Read the model definition and answer for the solid it produces. Units are mm, in the model's axes. A direction names the side the tool comes from. Coordinates: 2 decimals unless noted, no trailing zeros. Write each loop counter-clockwise with the first axis right and the second up, starting at its lowest first coordinate (ties: lowest second). Pieces come first, ordered by that corner, then holes. Notation, with made-up numbers: M 18.5,5.25 L 53.5,5.25 A18 ccw 53.5,39.25 Z; hole C 87.25,23 d7. An arc over 180 degrees is marked long. Write item = value, one per line.
from build123d import *

# Parameters (mm, degrees)
BOSS_EXTRUDE1_DEPTH = 14
SKETCH2_R           = 2
CUT_EXTRUDE1_DEPTH  = 20
SKETCH3_R           = 3.5
CUT_EXTRUDE2_DEPTH  = 3
SKETCH4_R           = 2.5
CUT_EXTRUDE3_DEPTH  = 8
FILLET1_R           = 0.5


with BuildPart() as part:
    # Sketch1 → Boss-Extrude1 (new body)
    with BuildSketch(Plane(origin=(0, 0, 0), x_dir=(1, 0, 0), z_dir=(0, 1, 0))):
        with BuildLine():
            Line((9, -14), (21, -14))
            Line((21, -14), (21, -20))
            Line((21, -20), (-21, -20))
            Line((-21, -20), (-21, -14))
            Line((-21, -14), (-9, -14))
            Line((-9, -14), (-9, 12.8))
            Line((-9, 12.8), (-1, 12.8))
            Line((-1, 12.8), (-1, 3.872983346))
            ThreePointArc((-1, 3.872983346), (0, -4), (1, 3.872983346))
            Line((1, 3.872983346), (1, 12.8))
            Line((1, 12.8), (9, 12.8))
            Line((9, 12.8), (9, -14))
        make_face()
    extrude(amount=BOSS_EXTRUDE1_DEPTH)

    # Sketch2 → Cut-Extrude1 (cut)
    with BuildSketch(Plane(origin=(9, 0, 0), x_dir=(0, 0, -1), z_dir=(1, 0, 0))):
        with Locations((8.3, 7)):
            Circle(SKETCH2_R)
    extrude(amount=-CUT_EXTRUDE1_DEPTH, mode=Mode.SUBTRACT)

    # Sketch3 → Cut-Extrude2 (cut)
    with BuildSketch(Plane(origin=(9, 0, 0), x_dir=(0, 0, -1), z_dir=(1, 0, 0))):
        with Locations((8.3, 7)):
            Circle(SKETCH3_R)
    extrude(amount=-CUT_EXTRUDE2_DEPTH, mode=Mode.SUBTRACT)

    # Sketch4 → Cut-Extrude3 (cut)
    with BuildSketch(Plane.XY.offset(20)):
        with Locations((-16, 7)):
            Circle(SKETCH4_R)
        with Locations((16, 7)):
            Circle(SKETCH4_R)
    extrude(amount=-CUT_EXTRUDE3_DEPTH, mode=Mode.SUBTRACT)

    # Fillet1
    fillet1_edges = [part.edges().sort_by_distance(p)[0] for p in [
        (-21, 7, 14),
        (-9, 7, 14),
        (-9, 7, -12.8),
        (9, 7, -12.8),
        (9, 7, 14),
        (21, 7, 14),
        (21, 7, 20),
        (-21, 7, 20),
    ]]
    fillet(fillet1_edges, radius=FILLET1_R)


solid = part.part
Item 1: Find section B-B (x = 16). Determine the outline of the cut face in (y, z).
Worked answers:
outline = M 0,14 L 4.5,14 L 4.5,20 L 0,20 Z; M 9.5,14 L 14,14 L 14,20 L 9.5,20 Z
Item 2: Consider line 1 along X through (y, z) = (4.75, 14.5); line 2 along Y through (x, z) = (16, 16.6); line 3 along X through (y, z) = (9, 12). Determine where each line is inside the solid, lowest interval first. Write a range as from..to.
Worked answers:
line_1 = -21..-17.09, -14.91..14.91, 17.09..21
line_2 = 0..4.5, 9.5..14
line_3 = -9..9
Item 3: For a pull along Y with two mould halves and no side action, classify faces 1 (the face through (0, 14, 11)), 2 (the face through (-14, 5, 14)), 3 (the face through (6, 5, -10)) as released by +Y, released by -Y, zero draft, split by the parting line, or undercut.
Worked answers:
face_1 = released by +Y
face_2 = zero draft
face_3 = undercut
Item 4: Find section A-A (z = -8.3). Determine the outline of the cut face in (x, y).
Worked answers:
outline = M -9,0 L -1,0 L -1,5 L -9,5 Z; M -9,9 L -1,9 L -1,14 L -9,14 Z; M 1,0 L 9,0 L 9,3.5 L 6,3.5 L 6,5 L 1,5 Z; M 1,9 L 6,9 L 6,10.5 L 9,10.5 L 9,14 L 1,14 Z
Item 5: Which of the six approach directions +Z, -Z, +X, -X, +Y, -Y give full straight-line access (tool end or side, diameter ignored) to faces 4 (the face through (1, 7, -6)), 5 (the face through (7.521, 3.895, -9.915)), 6 (the face through (9, 7, 0))?
Worked answers:
face_4 = -Z, +Y, -Y
face_5 = +X
face_6 = -Z, +X, +Y, -Y
Item 6: Find section C-C (z = 0). Determine the outline of the cut face in (x, y), and give its area (3 significant figures).
Worked answers:
outline = M -9,0 L -4,0 L -4,14 L -9,14 Z; M 4,0 L 9,0 L 9,14 L 4,14 Z
area = 140 mm²
Item 7: Flat-ended cylindrical pins translate along their axes: pin 1 (3.5 mm diameter, centred on y = 7, z = -8.3, fed in from +X); pin 2 (6 mm diameter, centred on y = 8, z = 1, fed in from -X); pin 3 (5.5 mm diameter, centred on x = 15, y = 7, fed in from -Z); pin 4 (3.5 mm diameter, centred on y = 7, z = -7.5, fed in from +X). Find the tip coordinate at first contact, or state that the pin passes through.
Worked answers:
pin_1 = through
pin_2 = -9
pin_3 = 14
pin_4 = 6
Item 8: Find section D-D (x = -7). Determine the outline of the cut face in (y, z), and give its area (3 significant figures).
Worked answers:
outline = M 0,-12.8 L 14,-12.8 L 14,20 L 0,20 Z; hole C 7,-8.3 d4
area = 447 mm²
